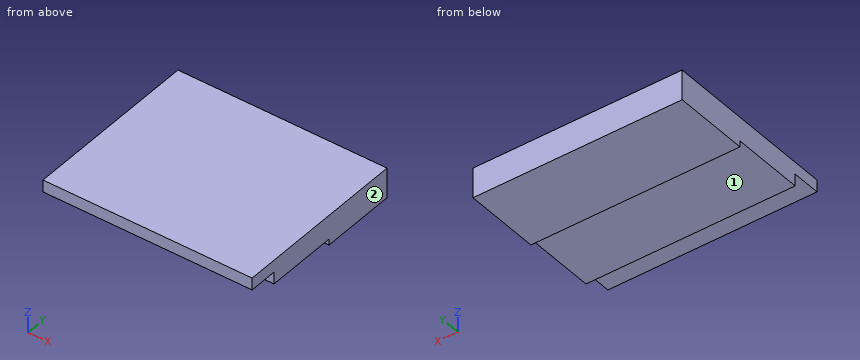
```python
from build123d import *

# Parameters (mm, degrees)
BOX041_W     = 174
BOX041_H     = 60.5
BOX041_DEPTH = 10
BOX042_W     = 174
BOX042_H     = 148
BOX042_DEPTH = 10
BOX040_W     = 174
BOX040_H     = 63.5
BOX040_DEPTH = 15


with BuildPart() as obj1:
    # Box041 → Box041 (new body)
    with BuildSketch(Plane(origin=(0, 21, 50), x_dir=(1, 0, 0), z_dir=(0, 0, 1))):
        with Locations((87, 30.25)):
            Rectangle(BOX041_W, BOX041_H)
    extrude(amount=BOX041_DEPTH)


with BuildPart() as obj2:
    # Box042 → Box042 (new body)
    with BuildSketch(Plane(origin=(0, -3, 60), x_dir=(1, 0, 0), z_dir=(0, 0, 1))):
        with Locations((87, 74)):
            Rectangle(BOX042_W, BOX042_H)
    extrude(amount=BOX042_DEPTH)


with BuildPart() as obj3:
    # Box040 → Box040 (new body)
    with BuildSketch(Plane(origin=(0, 81.5, 45), x_dir=(1, 0, 0), z_dir=(0, 0, 1))):
        with Locations((87, 31.75)):
            Rectangle(BOX040_W, BOX040_H)
    extrude(amount=BOX040_DEPTH)

    # Fusion010: union obj1, obj2
    add(obj1.part)
    add(obj2.part)


solid = obj3.part
```
Could you check a few things on this model? Use its own coordinates, in mm. Face numbers are marked on the shaded views. A direction names the side the tool comes from. Give positions to 0.01 mm unless a question says otherwise; leave off trailing zeros. Write each loop counter-clockwise with the first axis right and the second up, starting at its lowest first coordinate (ties: lowest second). Pieces come first, ordered by that corner, then holes. Notation, with made-up numbers: (19, -1.5) -> (37, -1.5) arc R27 ccw to (37, 15.5) -> close; hole circle Ø9 at (57.25, 64). An arc over 180 degrees is marked (long way). Write each question's results on one line, items separated by ' | '.
1. On a 3-axis mill with a long thin cutter (end or side, diameter ignored), from which of +Z, -Z, +X, -X, +Y, -Y can I reach the whole of each face in a straight line? I mean the marked faces 1 and 2. Say none if no direction works.
Check sheet entries:
face 1: -Z, +X, -X, -Y | face 2: +Z, -Z, +X, +Y, -Y
2. I want a section at C-C, the plane z = 55.75. Write out the boundary of the cut face in (x, y).
Check sheet entries:
outline: (0, 21) -> (174, 21) -> (174, 145) -> (0, 145) -> close
3. Will these pins go through, and if not, where does the flat tip stop? pin 1 Ø5 at (x, y) = (97.5, 37) entering from -Z; pin 2 Ø12 at (x, z) = (104.5, 48.5) entering from -Y; pin 3 Ø1.5 at (x, z) = (73, 47) entering from -Y.
Check sheet entries:
pin 1: stops at z = 50 | pin 2: stops at y = 21 | pin 3: stops at y = 81.5
4. I want a section at A-A, the plane x = 68. Write out the boundary of the cut face in (y, z).
Check sheet entries:
outline: (-3, 60) -> (21, 60) -> (21, 50) -> (81.5, 50) -> (81.5, 45) -> (145, 45) -> (145, 70) -> (-3, 70) -> close
5. I want a section at B-B, the plane y = 54.5. Write out the boundary of the cut face in (x, z), then the cut area to 3 significant figures.
Check sheet entries:
outline: (0, 50) -> (174, 50) -> (174, 70) -> (0, 70) -> close | area: 3,480 mm²
6. I need wall thicknesses on L1, parallel to Z at x = 51, y = 43.5; L2, parallel to Z at x = 47.5, y = 7; L3, parallel to Y at x = 11, z = 59.25. Which ranges of each line are inside material? Lowest first, please.
Check sheet entries:
L1: z = 50 to 70 | L2: z = 60 to 70 | L3: y = 21 to 145
